```python
from build123d import *

# Parameters (mm, degrees)
F0_W     = 381.508
F0_H     = 236.728
F1_DEPTH = 5


with BuildPart() as f1:
    # F0 (on Front) → F1 (new body)
    with BuildSketch(Plane.XZ):
        with Locations((2.340291, -78.132914)):
            Rectangle(F0_W, F0_H)
        Polygon((-180.793709, -180.748914), (-180.793709, 26.261086), (-160.473709, 26.261086), (-160.473709, 32.357086), (-147.265709, 32.357086), (-147.265709, 26.261086), (145.088291, 26.261086), (145.088291, 32.357086), (158.296291, 32.357086), (158.296291, 26.261086), (178.616291, 26.261086), (178.616291, -180.748914), (159.515491, -180.748914), (159.515491, -187.987914), (144.402491, -187.987914), (144.402491, -180.748914), (141.075091, -180.748914), (141.075091, -190.786994), (-141.245909, -190.786994), (-141.245909, -180.748914), (-146.579909, -180.748914), (-146.579909, -187.987914), (-161.692909, -187.987914), (-161.692909, -180.748914), align=None, mode=Mode.SUBTRACT)
    extrude(amount=F1_DEPTH)


solid = f1.part
```
CAD build for the part. Positions are in the model's coordinates, mm. Round coordinates to 2 decimals unless told otherwise and drop trailing zeros. Write each loop counter-clockwise with the first axis right and the second up, starting at its lowest first coordinate (ties: lowest second). Pieces come first, ordered by that corner, then holes. Notation, with made-up numbers: (15.5, 54) - (66.5, 54) arc R27 cw to (66.5, 86) - close; hole circle Ø7 at (75, -2). An arc over 180 degrees is marked (long way). Write item = value, one per line. Start each with the question number.
Q1. Band-saw the part on A-A (x = 111). Give the cut face in (y, z), then the cut area to 3 significant figures.
Q2. Band-saw the part on C-C (y = -2.9). Give the cut face in (x, z).
Q3. Band-saw the part on B-B (z = -76.5). Give the cut face in (x, y).
Q4. Probe L1, parallel to Z at x = -125.5, y = -4.05; L2, parallel to X at y = -1.5, z = -149.5; L3, parallel to Z at x = -143.5, y = -3.4. List the from-to ranges inside material, lowest first. Write a range as from..to.
Answers below:
q1.outline = (-5, -196.5) - (0, -196.5) - (0, -190.79) - (-5, -190.79) - close; (-5, 26.26) - (0, 26.26) - (0, 40.23) - (-5, 40.23) - close
q1.area = 98.4 mm2
q2.outline = (-188.41, -196.5) - (193.09, -196.5) - (193.09, 40.23) - (-188.41, 40.23) - close; hole (-180.79, -180.75) - (-161.69, -180.75) - (-161.69, -187.99) - (-146.58, -187.99) - (-146.58, -180.75) - (-141.25, -180.75) - (-141.25, -190.79) - (141.08, -190.79) - (141.08, -180.75) - (144.4, -180.75) - (144.4, -187.99) - (159.52, -187.99) - (159.52, -180.75) - (178.62, -180.75) - (178.62, 26.26) - (158.3, 26.26) - (158.3, 32.36) - (145.09, 32.36) - (145.09, 26.26) - (-147.27, 26.26) - (-147.27, 32.36) - (-160.47, 32.36) - (-160.47, 26.26) - (-180.79, 26.26) - close
q3.outline = (-188.41, -5) - (-180.79, -5) - (-180.79, 0) - (-188.41, 0) - close; (178.62, -5) - (193.09, -5) - (193.09, 0) - (178.62, 0) - close
q4.L1 = -196.5..-190.79, 26.26..40.23
q4.L2 = -188.41..-180.79, 178.62..193.09
q4.L3 = -196.5..-180.75, 26.26..40.23
